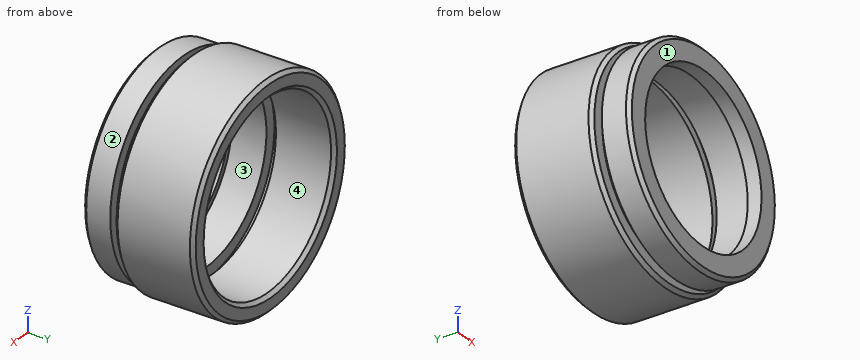
from build123d import *

# Parameters (mm, degrees)
CHAMFER_1_SIZE = 0.5


with BuildPart() as part:
    # 草图1 → 旋转1 (revolve)
    with BuildSketch(Plane.XY, mode=Mode.PRIVATE) as revolve_1_sk:
        Polygon((12, 0), (15.25, 0), (15.25, 4), (13.75, 4), (13.75, 5), (15.875, 5), (15.875, 16.5), (13.25, 16.5), (13.25, 8), (14.35, 8), (14.35, 7), (12.7, 7), (12.7, 2), (12, 2), align=None)
    revolve(revolve_1_sk.sketch.rotate(Axis((0, 0, 0), (0, 1, 0)), 90), axis=Axis((0, 0, 0), (0, 1, 0)))  # turned: the seam where the file's is

    # 倒角1
    chamfer_1_edges = [part.edges().sort_by_distance(p)[0] for p in [
        (0, 16.5, 13.25),
        (0, 16.5, 15.875),
        (0, 5, 15.875),
        (0, 0, 15.25),
    ]]
    chamfer(chamfer_1_edges, length=CHAMFER_1_SIZE)


solid = part.part
Check sheet for the modelled part. Datum: model origin and axes. Units: mm. Face numbers are marked on the shaded views. Give positions to 0.01 mm unless a question says otherwise; leave off trailing zeros. Write each loop counter-clockwise with the first axis right and the second up, starting at its lowest first coordinate (ties: lowest second). Pieces come first, ordered by that corner, then holes. Notation, with made-up numbers: (45.5, 60) -> (79.5, 60) arc R16 ccw to (79.5, 87) -> close; hole circle Ø6 at (34, 80). An arc over 180 degrees is marked (long way). One line per item, written item: value. Start each with the question number.
Item 1: Section check B-B on y = 2.5. Record the cut outline in (x, z).
Item 2: Gauge pin test, flat ends, axial feed: pin 1 (3 mm diameter, centred on x = -6, y = 10, fed in from -Z); pin 2 (5 mm diameter, centred on y = 6, z = 8, fed in from +X); pin 3 (19 mm diameter, centred on x = 0, z = 0, fed in from -Y); pin 4 (6 mm diameter, centred on y = 5.5, z = 12, fed in from -X). Record the tip position at first contact, or that the pin passes through.
Item 3: Draft check along Z on the marked faces 1, 2, 3 and 4. Enter one of: +Z half, -Z half, draft (parallel to the pull), parting line (faces both ways), or undercut.
Item 4: Material ranges on probe 1 along X at (y, z) = (3.2, 0); probe 2 along X at (y, z) = (12, 0) (3 decimals); probe 3 along Y at (x, z) = (-4.5, 14), recorded low to high. Write a range as from..to.
Item 5: Section check A-A on y = 7.5. Record the cut outline in (x, z) (3 decimals), then the cut area to 3 significant figures.
Results list:
1. outline: circle Ø30.5 at (0, 0); hole circle Ø25.4 at (0, 0)
2. pin 1: z = -15.22
2. pin 2: x = 14.89
2. pin 3: through
2. pin 4: x = -13.08
3. face 1: draft
3. face 2: parting line
3. face 3: undercut
3. face 4: undercut
4. probe 1: -15.25..-12.7, 12.7..15.25
4. probe 2: -15.875..-13.25, 13.25..15.875
4. probe 3: 0..4, 5..16.5
5. outline: circle Ø31.75 at (0, 0); hole circle Ø28.7 at (0, 0)
5. area: 145 mm²
